from build123d import *

# Parameters (mm, degrees)
BOSS_EXTRUDE1_DEPTH      = 20
M3_CLEARANCE_HOLE1_D     = 3.4
M3_CLEARANCE_HOLE1_DEPTH = 12
M3_CLEARANCE_HOLE1_TIP   = 1.021463052
SKETCH5_R                = 1.5
BOSS_EXTRUDE2_DEPTH      = 8


with BuildPart() as part:
    # Sketch1 → Boss-Extrude1 (new body)
    with BuildSketch(Plane(origin=(0, 0, 0), x_dir=(1, 0, 0), z_dir=(0, 1, 0))):
        Polygon((3.175426481, 0), (1.58771324, 2.75), (-1.58771324, 2.75), (-3.175426481, 0), (-1.58771324, -2.75), (1.58771324, -2.75), align=None)
    extrude(amount=BOSS_EXTRUDE1_DEPTH)

    # M3 Clearance Hole1
    with Locations(Plane(origin=(0, 20, 0), x_dir=(-1, 0, 0), z_dir=(0, 1, 0))):
        with Locations((0, 0)):
            Hole(M3_CLEARANCE_HOLE1_D / 2, depth=M3_CLEARANCE_HOLE1_DEPTH)
            with Locations((0, 0, -(M3_CLEARANCE_HOLE1_DEPTH + M3_CLEARANCE_HOLE1_TIP / 2))):  # 118° drill point
                Cone(0, M3_CLEARANCE_HOLE1_D / 2, M3_CLEARANCE_HOLE1_TIP, mode=Mode.SUBTRACT)

    # Sketch4 → Cut-Revolve1 (revolve, cut)
    with BuildSketch(Plane.XY):
        with BuildLine():
            Line((-2.175426481, 20), (-3.175426481, 20))
            Line((-3.175426481, 20), (-3.175426481, 19))
            ThreePointArc((-3.175426481, 19), (-2.882533262, 19.707106781), (-2.175426481, 20))
        make_face()
        with BuildLine():
            Line((-3.175426481, 1), (-3.175426481, 0))
            Line((-3.175426481, 0), (-2.175426481, 0))
            ThreePointArc((-2.175426481, 0), (-2.882533262, 0.292893219), (-3.175426481, 1))
        make_face()
    revolve(axis=Axis((0, 20, 0), (0, -1, 0)), mode=Mode.SUBTRACT)

    # Sketch5 → Boss-Extrude2 (add)
    with BuildSketch(Plane.XZ):
        Circle(SKETCH5_R)
    extrude(amount=BOSS_EXTRUDE2_DEPTH)


solid = part.part
Verification items for the finished model (mm, model axes). A direction names the side the tool comes from. Coordinates: 2 decimals unless noted, no trailing zeros. Order: outer loops, then holes, each group sorted by start corner. A loop starts at its lowest first (then second) coordinate and runs counter-clockwise, first axis right, second up.
1. Scan lines: line 1 (Z direction, x = 0, y = 15); line 2 (Y direction, x = 0, z = -1.75); line 3 (X direction, y = 9.5, z = 2.15). Record each from-to range of solid material in increasing order.
Results found:
line 1: z = -2.75 to -1.7, 1.7 to 2.75
line 2: y = 0 to 20
line 3: x = -1.93 to 1.93
2. Set-up check for faces 4 (the face through (0, 20, 2)), 5 (the face through (-1.5, -3.94, 0.07)): record each of +Z, -Z, +X, -X, +Y, -Y from which the full face is reachable in a straight line by a thin tool's end or side.
Results found:
face 4: +Z, -Z, +X, -X, +Y
face 5: -Y
3. Sectioned sample at B-B, the plane y = 2. Record the cut outline in (x, z), and give its area (3 significant figures).
Results found:
outline: (-3.18, 0) - (-1.59, -2.75) - (1.59, -2.75) - (3.18, 0) - (1.59, 2.75) - (-1.59, 2.75) - close
area: 26.2 mm2
4. Sectioned sample at A-A, the plane y = 9.5. Record the cut outline in (x, z).
Results found:
outline: (-3.18, 0) - (-1.59, -2.75) - (1.59, -2.75) - (3.18, 0) - (1.59, 2.75) - (-1.59, 2.75) - close; hole circle Ø3.4 at (0, 0)
5. Release check for a two-part mould opening along X. For faces 1 (the face through (-0.37, 13.92, -1.66)), 2 (the face through (2.37, 9.863, 1.394)), 3 (the face through (0, -8, 0)) record: +X half, -X half, draft (parallel to the pull), parting line (faces both ways), or undercut.
Results found:
face 1: undercut
face 2: +X half
face 3: draft
